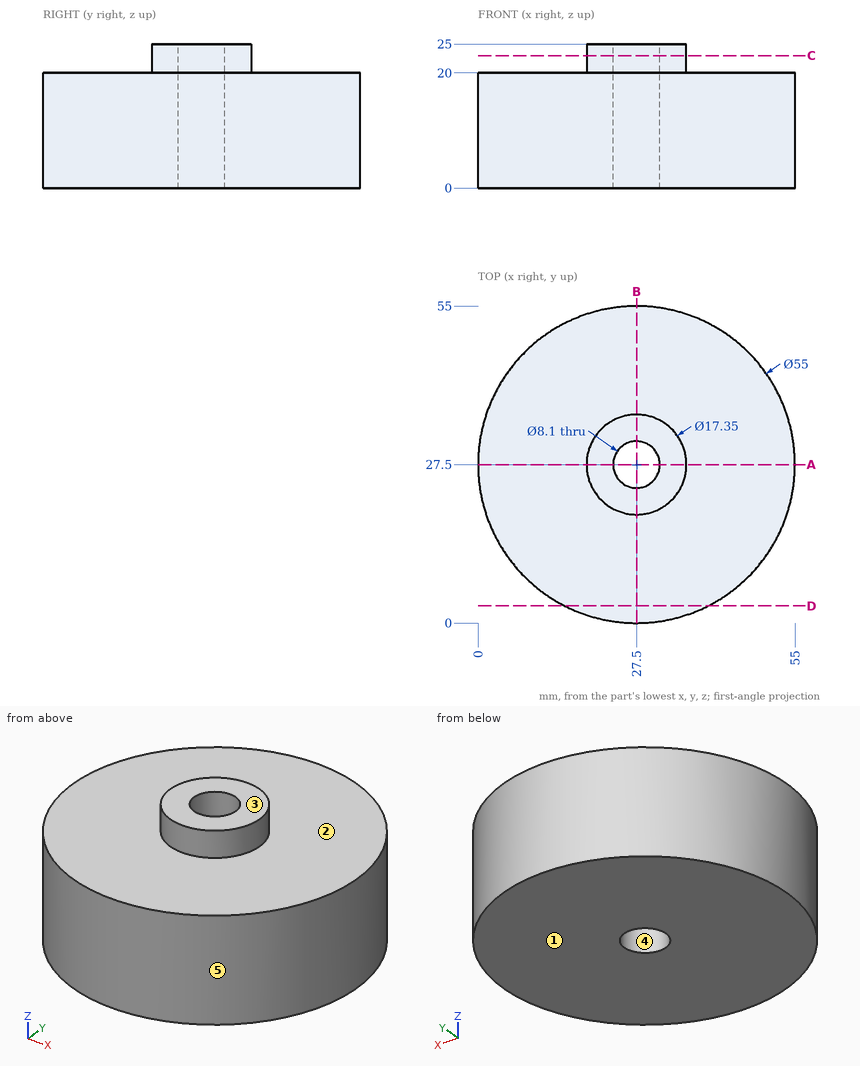
Job drawing, mm, ordinate dimensions from the low corner. One solid piece. A direction names the side the tool comes from. Coordinates: 2 decimals unless noted, no trailing zeros. Loops run counter-clockwise (first coordinate to the right, second up) from the corner with the lowest first, then second, coordinate; pieces in that order, holes last. Notation, with made-up numbers: (-5, 65.5) - (18, 65.5) arc R22 cw to (18, 79.5) - close; hole circle Ø3 at (72, 36). An arc over 180 degrees is marked (long way). Write item = value, one per line. Start each with the question number.
Q1. Pull direction X, two halves, no side cores. Call the marked faces 3, 4 and 5: pulls with the +X half, pulls with the -X half, needs draft (parallel to the pull), parting line crosses it, or undercut.
Q2. Drill centre lines: L1, parallel to Y at x = 27.5, z = 16.25; L2, parallel to Z at x = 50, y = 19; L3, parallel to X at y = 23, z = 11.5. Where is each one in solid material? Low to high.
Q3. Cut at C-C, the plane z = 23. List the corners of the cut face in (x, y) (3 decimals), then the cut area to 3 significant figures.
Q4. Flat gauge pins, fed straight in: pin 1 Ø4 at (x, z) = (27.5, 15.5) entering from +Y; pin 2 Ø1 at (y, z) = (26, 8) entering from -X; pin 3 Ø1.5 at (x, z) = (10.5, 17.5) entering from +Y; pin 4 Ø1.5 at (x, y) = (34.5, 21.5) entering from +Z. Where does each tip first touch, or does it go through?
Q5. Cut at A-A, the plane y = 27.5. List the corners of the cut face in (x, z) (3 decimals).
Q6. Which spindle directions (+Z, -Z, +X, -X, +Y, -Y) get a long thin tool onto all of the face, cutting with end or side? Do the marked faces 1 and 2. Say none if no direction does.
Q7. Cut at D-D, the plane y = 3. List the corners of the cut face in (x, z).
Computed:
q1.face_3 = needs draft
q1.face_4 = undercut
q1.face_5 = parting line crosses it
q2.L1 = 0 to 23.45, 31.55 to 55
q2.L2 = 0 to 20
q2.L3 = 0.37 to 54.63
q3.outline = circle Ø17.35 at (27.5, 27.5); hole circle Ø8.1 at (27.5, 27.5)
q3.area = 185 mm²
q4.pin_1 = 55
q4.pin_2 = 0.02
q4.pin_3 = 49.69
q4.pin_4 = 25
q5.outline = (0, 0) - (23.45, 0) - (23.45, 25) - (18.825, 25) - (18.825, 20) - (0, 20) - close; (31.55, 0) - (55, 0) - (55, 20) - (36.175, 20) - (36.175, 25) - (31.55, 25) - close
q6.face_1 = -Z, +X, -X, +Y, -Y
q6.face_2 = +Z
q7.outline = (15.01, 0) - (39.99, 0) - (39.99, 20) - (15.01, 20) - close
